from build123d import *

# Parameters (mm, degrees)
F0_W     = 63.5
F0_H     = 63.5
F1_DEPTH = 63.5
F2_R     = 19.05
F3_DEPTH = 38.1
F4_R     = 19.05
F5_DEPTH = 38.1


with BuildPart() as f1:
    # F0 (on Front) → F1 (new body)
    with BuildSketch(Plane.XZ):
        with Locations((31.75, 31.75)):
            Rectangle(F0_W, F0_H)
    extrude(amount=F1_DEPTH)

    # F2 (on Top) → F3 (join)
    with BuildSketch(Plane.XY):
        Circle(F2_R)
    extrude(amount=F3_DEPTH)

    # F4 (on Top) → F5 (join)
    with BuildSketch(Plane.XY):
        Circle(F4_R)
    extrude(amount=F5_DEPTH)


solid = f1.part
CAD build for the part. Positions are in the model's coordinates, mm. A direction names the side the tool comes from. Coordinates: 2 decimals unless noted, no trailing zeros. Order: outer loops, then holes, each group sorted by start corner. A loop starts at its lowest first (then second) coordinate and runs counter-clockwise, first axis right, second up. Notation, with made-up numbers: (-31, 41) -> (1, 41) arc R21 ccw to (1, 52) -> close; hole circle Ø6 at (55.5, 10.5). An arc over 180 degrees is marked (long way). Answer in a Markdown table with one row per item.
1) Band-saw the part on D-D (y = -55.5). List the corners of the cut face in (x, z).
Check values:
| item | result |
|---|---|
| outline | (0, 0) -> (63.5, 0) -> (63.5, 63.5) -> (0, 63.5) -> close |
2) Band-saw the part on A-A (z = 4.5). List the corners of the cut face in (x, y).
Check values:
| item | result |
|---|---|
| outline | (0, -63.5) -> (63.5, -63.5) -> (63.5, 0) -> (19.05, 0) arc R19.05 ccw (long way) to (0, -19.05) -> close |
3) Flat gauge pins, fed straight in: P1, Ø10, axis at x = 22.5, z = 7, coming from the +Y side; P2, Ø1.5, axis at x = 17, y = -11, coming from the -Z side; P3, Ø19, axis at x = 43, z = 18, coming from the +Y side; P4, Ø4, axis at x = -7, y = -0.5, coming from the +Z side. Where does each tip first touch, or does it go through?
Check values:
| item | result |
|---|---|
| P1 | y = 7.53 |
| P2 | z = 0 |
| P3 | y = 0 |
| P4 | z = 38.1 |
4) Which spindle directions (+Z, -Z, +X, -X, +Y, -Y) get a long thin tool onto all of the face, cutting with end or side? Do faces 1 (the face through (0, -38, 31)), 2 (the face through (38, 0, 32)), 3 (the face through (31, -63.5, 32)). Say none if no direction does.
Check values:
| item | result |
|---|---|
| face 1 | +Z, -X, -Y |
| face 2 | +Z, +X, +Y |
| face 3 | +Z, -Z, +X, -X, -Y |
5) Band-saw the part on C-C (x = 21). List the corners of the cut face in (y, z), and give its area (3 significant figures).
Check values:
| item | result |
|---|---|
| outline | (-63.5, 0) -> (0, 0) -> (0, 63.5) -> (-63.5, 63.5) -> close |
| area | 4,030 mm2 |
6) Band-saw the part on B-B (y = -2). List the corners of the cut face in (x, z), and give its area (3 significant figures).
Check values:
| item | result |
|---|---|
| outline | (-18.94, 0) -> (63.5, 0) -> (63.5, 63.5) -> (0, 63.5) -> (0, 38.1) -> (-18.94, 38.1) -> close |
| area | 4,750 mm2 |
7) Drill centre lines: line 1 (X direction, y = -26, z = 60.5); line 2 (Y direction, x = 22, z = 53); line 3 (Z direction, x = -1.5, y = -5). Where is each one in solid material? Low to high.
Check values:
| item | result |
|---|---|
| line 1 | 0 to 63.5 |
| line 2 | -63.5 to 0 |
| line 3 | 0 to 38.1 |
